from build123d import *

# Parameters (mm, degrees)
SKETCH_1_W             = 21
SKETCH_1_H             = 15
EXTRUDE_1_DEPTH        = 17
SKETCH_3_OUTSIDE_W     = 29.18
SKETCH_3_OUTSIDE_H     = 23.18
SKETCH_3_OUTSIDE_W_2   = 18
SKETCH_3_OUTSIDE_H_2   = 12
CUT_EXTRUDE_1_DEPTH    = 11
SKETCH_4_OUTSIDE_W     = 29.18
SKETCH_4_OUTSIDE_H     = 23.18
SKETCH_4_OUTSIDE_W_2   = 15
SKETCH_4_OUTSIDE_H_2   = 9
CUT_EXTRUDE_2_DEPTH    = 4
CUT_EXTRUDE_3_REACH    = 14
CUT_EXTRUDE_4_REACH    = 14
FILLET_2_R             = 0.2
CHAMFER_1_SIZE         = 1
CHAMFER_1_SIZE2        = 1.732050808
CHAMFER_1_PART_2_SIZE  = 1
CHAMFER_1_PART_2_SIZE2 = 1.732050808
CHAMFER_1_PART_3_SIZE  = 1
CHAMFER_1_PART_3_SIZE2 = 1.732050808
CHAMFER_1_PART_4_SIZE  = 1
CHAMFER_1_PART_4_SIZE2 = 1.732050808
CUT_EXTRUDE_5_REACH    = 15.5
SKETCH_7_W             = 3.215432019
SKETCH_7_H             = 8
SKETCH_8_W             = 0.5
SKETCH_8_H             = 6
EXTRUDE_2_DEPTH        = 1.6
EXTRUDE_3_DEPTH        = 8
PATTERN_LINEAR_2_COUNT = 3
PATTERN_LINEAR_2_PITCH = 7
PATTERN_LINEAR_3_COUNT = 2
PATTERN_LINEAR_3_PITCH = 7


with BuildPart() as part:
    # 草图1 → 凸台-拉伸1 (new body)
    with BuildSketch(Plane.XY):
        with Locations((10.5, 7.5)):
            Rectangle(SKETCH_1_W, SKETCH_1_H)
    extrude(amount=EXTRUDE_1_DEPTH)

    # 草图3 outside → 切除-拉伸1 (cut)
    with BuildSketch(Plane(origin=(0, 0, 0), x_dir=(-1, 0, 0), z_dir=(0, 0, -1))):
        with Locations((-10.5, 7.5)):
            Rectangle(SKETCH_3_OUTSIDE_W, SKETCH_3_OUTSIDE_H)
        with Locations((-10.5, 7.5)):
            Rectangle(SKETCH_3_OUTSIDE_W_2, SKETCH_3_OUTSIDE_H_2, mode=Mode.SUBTRACT)
    extrude(amount=-CUT_EXTRUDE_1_DEPTH, mode=Mode.SUBTRACT)

    # 草图4 outside → 切除-拉伸2 (cut)
    with BuildSketch(Plane.XY.offset(17)):
        with Locations((10.5, 7.5)):
            Rectangle(SKETCH_4_OUTSIDE_W, SKETCH_4_OUTSIDE_H)
        with Locations((10.5, 7.5)):
            Rectangle(SKETCH_4_OUTSIDE_W_2, SKETCH_4_OUTSIDE_H_2, mode=Mode.SUBTRACT)
    extrude(amount=-CUT_EXTRUDE_2_DEPTH, mode=Mode.SUBTRACT)

    # 草图5 → 切除-拉伸3 (cut, up to next)
    with BuildSketch(Plane.XZ.offset(-3), mode=Mode.PRIVATE) as cut_extrude_3_sk1:
        with BuildLine():
            Line((3, 17), (3.786081295, 18.926671419))
            Line((3.786081295, 18.926671419), (19.848042348, 18.643435221))
            Line((19.848042348, 18.643435221), (18, 13))
            ThreePointArc((18, 13), (10.37304874, 14.523932773), (3, 17))
        make_face()
    cut_extrude_3_tool1 = extrude(cut_extrude_3_sk1.sketch, amount=-CUT_EXTRUDE_3_REACH, mode=Mode.PRIVATE) & part.part
    add(cut_extrude_3_tool1.solids().sort_by_distance((12.266887, 3, 16.568518))[0], mode=Mode.SUBTRACT)

    # 草图6 → 切除-拉伸4 (cut, up to next)
    with BuildSketch(Plane.XZ.offset(-3), mode=Mode.PRIVATE) as cut_extrude_4_sk1:
        with BuildLine():
            Line((3.538726555, 16.783166359), (1.834472807, 18.259535343))
            Line((1.834472807, 18.259535343), (1.834472807, 13.545763946))
            Line((1.834472807, 13.545763946), (3, 13))
            ThreePointArc((3, 13), (3.102200266, 14.915387354), (3.538726555, 16.783166359))
        make_face()
    cut_extrude_4_tool1 = extrude(cut_extrude_4_sk1.sketch, amount=-CUT_EXTRUDE_4_REACH, mode=Mode.PRIVATE) & part.part
    add(cut_extrude_4_tool1.solids().sort_by_distance((2.498394, 3, 15.595743))[0], mode=Mode.SUBTRACT)

    # 圆角2
    fillet_2_edges = [part.edges().sort_by_distance(p)[0] for p in [
        (3.538726555, 7.5, 16.783166359),
    ]]
    fillet(fillet_2_edges, radius=FILLET_2_R)

    # 倒角1
    chamfer_1_edges = [part.edges().sort_by_distance(p)[0] for p in [
        (10.5, 15, 13),
    ]]
    chamfer_1_side = [part.faces().sort_by_distance(p)[0] for p in [
        (10.5, 15, 12),
    ]]
    chamfer(chamfer_1_edges, length=CHAMFER_1_SIZE, length2=CHAMFER_1_SIZE2, reference=chamfer_1_side[0])

    # 倒角1 part 2
    chamfer_1_part_2_edges = [part.edges().sort_by_distance(p)[0] for p in [
        (0, 7.5, 13),
    ]]
    chamfer_1_part_2_side = [part.faces().sort_by_distance(p)[0] for p in [
        (0, 7.5, 12),
    ]]
    chamfer(chamfer_1_part_2_edges, length=CHAMFER_1_PART_2_SIZE, length2=CHAMFER_1_PART_2_SIZE2, reference=chamfer_1_part_2_side[0])

    # 倒角1 part 3
    chamfer_1_part_3_edges = [part.edges().sort_by_distance(p)[0] for p in [
        (10.5, 0, 13),
    ]]
    chamfer_1_part_3_side = [part.faces().sort_by_distance(p)[0] for p in [
        (10.5, 0, 12),
    ]]
    chamfer(chamfer_1_part_3_edges, length=CHAMFER_1_PART_3_SIZE, length2=CHAMFER_1_PART_3_SIZE2, reference=chamfer_1_part_3_side[0])

    # 倒角1 part 4
    chamfer_1_part_4_edges = [part.edges().sort_by_distance(p)[0] for p in [
        (21, 7.5, 13),
    ]]
    chamfer_1_part_4_side = [part.faces().sort_by_distance(p)[0] for p in [
        (21, 7.5, 12),
    ]]
    chamfer(chamfer_1_part_4_edges, length=CHAMFER_1_PART_4_SIZE, length2=CHAMFER_1_PART_4_SIZE2, reference=chamfer_1_part_4_side[0])

    # 草图7 → 切除-拉伸5 (cut, up to next)
    with BuildSketch(Plane.XZ.offset(-1.5), mode=Mode.PRIVATE) as cut_extrude_5_sk1:
        with Locations((0.39228399, 7)):
            Rectangle(SKETCH_7_W, SKETCH_7_H)
    cut_extrude_5_tool1 = extrude(cut_extrude_5_sk1.sketch, amount=-CUT_EXTRUDE_5_REACH, mode=Mode.PRIVATE) & part.part
    add(cut_extrude_5_tool1.solids().sort_by_distance((0.392284, 1.5, 7))[0], mode=Mode.SUBTRACT)
    # 草图7 → 切除-拉伸5 (cut, up to next)
    with BuildSketch(Plane.XZ.offset(-1.5), mode=Mode.PRIVATE) as cut_extrude_5_sk2:
        with Locations((20.60771601, 7)):
            Rectangle(SKETCH_7_W, SKETCH_7_H)
    cut_extrude_5_tool2 = extrude(cut_extrude_5_sk2.sketch, amount=-CUT_EXTRUDE_5_REACH, mode=Mode.PRIVATE) & part.part
    add(cut_extrude_5_tool2.solids().sort_by_distance((20.607716, 1.5, 7))[0], mode=Mode.SUBTRACT)

    # 扫描1: sweep along a path in 草图9
    with BuildLine(Plane(origin=(0, 7.5, 0), x_dir=(-1, 0, 0), z_dir=(0, -1, 0))) as sweep_1_path:
        Line((-1.75, -3), (-0.309821019, -6.95685923))
        ThreePointArc((-0.309821019, -6.95685923), (-0.195012991, -7.793192673), (-0.4354877, -8.602393776))
        Line((-0.4354877, -8.602393776), (-1.75, -11))
    # 草图8 → 扫描1 (sweep)
    with BuildSketch(Plane.XY.offset(3)):
        with Locations((1.75, 7.5)):
            Rectangle(SKETCH_8_W, SKETCH_8_H)
    sweep_1 = sweep(path=sweep_1_path.line)

    # 镜向1: 扫描1 across plane
    add(sweep_1.mirror(Plane(origin=(10.5, 0, 0), x_dir=(0, 0, 1), z_dir=(1, 0, 0))))

    # 草图10 → 凸台-拉伸2 (add)
    with BuildSketch(Plane(origin=(0, 0, 0), x_dir=(-1, 0, 0), z_dir=(0, 0, -1))):
        with BuildLine():
            Line((-5, 5), (-5, 10))
            ThreePointArc((-5, 10), (-3.5, 11.5), (-2, 10))
            Line((-2, 10), (-2, 5))
            ThreePointArc((-2, 5), (-3.5, 3.5), (-5, 5))
        make_face()
    extrude_2 = extrude(amount=EXTRUDE_2_DEPTH)

    # 草图11 → 凸台-拉伸3 (add)
    with BuildSketch(Plane(origin=(0, 0, -1.6), x_dir=(-1, 0, 0), z_dir=(0, 0, -1))):
        with BuildLine():
            Line((-4, 6), (-4, 9))
            ThreePointArc((-4, 9), (-3.5, 9.5), (-3, 9))
            Line((-3, 9), (-3, 6))
            ThreePointArc((-3, 6), (-3.5, 5.5), (-4, 6))
        make_face()
    extrude_3 = extrude(amount=EXTRUDE_3_DEPTH)

    # 阵列(线性)2: 凸台-拉伸2 ×3
    with Locations(*[(i * PATTERN_LINEAR_2_PITCH, 0, 0) for i in range(1, PATTERN_LINEAR_2_COUNT)]):
        add(extrude_2)

    # 阵列(线性)3: 凸台-拉伸3 ×2
    with Locations(*[(i * PATTERN_LINEAR_3_PITCH, 0, 0) for i in range(1, PATTERN_LINEAR_3_COUNT)]):
        add(extrude_3)


solid = part.part
Part model, mm, in its own coordinate system. A direction names the side the tool comes from. Give positions to 0.01 mm unless a question says otherwise; leave off trailing zeros. Order: outer loops, then holes, each group sorted by start corner. A loop starts at its lowest first (then second) coordinate and runs counter-clockwise, first axis right, second up. Notation, with made-up numbers: (-3.75, -7.5) -> (12.25, -7.5) arc R6 ccw to (12.25, -2.5) -> close; hole circle Ø2 at (59.25, 38). An arc over 180 degrees is marked (long way). Use one line per item in the form item = value.
(1) Pull direction Z, two halves, no side cores. Call faces 6 (the face through (10.4, 15, 11.5)), 7 (the face through (4.15, 7.56, -1.6)), 8 (the face through (20.6, 4.5, 6.7)): +Z half, -Z half, draft (parallel to the pull), parting line (faces both ways), or undercut.
Solution:
face_6 = draft
face_7 = -Z half
face_8 = undercut
(2) Saw through at B-B (z = 10.5). Write the cut outline in (x, y), then the cut area to 3 significant figures.
Solution:
outline = (1.21, 4.5) -> (1.74, 4.5) -> (1.74, 10.5) -> (1.21, 10.5) -> close; (2, 1.5) -> (19, 1.5) -> (19, 13.5) -> (2, 13.5) -> close; (19.26, 4.5) -> (19.79, 4.5) -> (19.79, 10.5) -> (19.26, 10.5) -> close
area = 210 mm²
(3) Saw through at D-D (y = 1). Write the cut outline in (x, z), then the cut area to 3 significant figures.
Solution:
outline = (0, 11) -> (21, 11) -> (21, 12) -> (20, 12.58) -> (1, 12.58) -> (0, 12) -> close
area = 32.5 mm²
(4) Saw through at A-A (z = -3). Write the cut outline in (x, y), then the cut area to 3 significant figures.
Solution:
outline = (3, 6) arc R0.5 ccw to (4, 6) -> (4, 9) arc R0.5 ccw to (3, 9) -> close; (10, 6) arc R0.5 ccw to (11, 6) -> (11, 9) arc R0.5 ccw to (10, 9) -> close
area = 7.57 mm²
(5) Drill centre lines: line 1 (X direction, y = 1.25, z = 11.5); line 2 (Z direction, x = 17.25, y = 13.25); line 3 (Y direction, x = 16.75, z = 8.75). Where is each one in solid material? Low to high. Write a range as from..to.
Solution:
line_1 = 0..21
line_2 = 0..13
line_3 = 1.5..13.5
(6) Flat gauge pins, fed straight in: P1, Ø2.5, axis at y = 7, z = -6.5, coming from the -X side; P2, Ø3, axis at x = 19, y = 12.5, coming from the -Z side; P3, Ø3, axis at x = 13.5, y = 11.5, coming from the +Z side; P4, Ø4, axis at y = 5, z = 7.5, coming from the +X side. Where does each tip first touch, or does it go through?
Solution:
P1 = 3
P2 = -1.6
P3 = 14.11
P4 = 21.05
(7) Tool access for faces 1 (the face through (11, 7, -6)), 2 (the face through (11, 13.5, 5)), 3 (the face through (10.5, 5.5, -5.5)), 4 (the face through (21, 7.4, 11.5)), 5 (the face through (12, 7, -1)): list every direction of +Z, -Z, +X, -X, +Y, -Y with a clear straight run to the whole face (end or side of a thin tool).
Solution:
face_1 = -Z, +X, +Y, -Y
face_2 = -Z, +X, -X, +Y
face_3 = -Z, -Y
face_4 = +Z, +X, +Y, -Y
face_5 = -Z, +Y, -Y
(8) Saw through at C-C (x = 6.5). Write the cut outline in (y, z).
Solution:
outline = (0, 11) -> (1.5, 11) -> (1.5, 0) -> (13.5, 0) -> (13.5, 11) -> (15, 11) -> (15, 12) -> (13.27, 13) -> (12, 13) -> (12, 15.69) -> (3, 15.69) -> (3, 13) -> (1.73, 13) -> (0, 12) -> close
